from build123d import *

# Parameters (mm, degrees)
F1_DEPTH  = 6.35
F2_R      = 46.355
F2_R_2    = 8.1788
F2_R_3    = 10.16
F2_R_4    = 3.175
F2_R_5    = 3.556
F2_R_6    = 2.38125
F3_DEPTH  = 6.351
F4_R      = 48.895
F5_DEPTH  = 2.413
F6_SIZE   = 0.79375
F7_R      = 6.731
F7_R_2    = 7.1501
F8_DEPTH  = 3.96875
F9_R      = 3.571875
F10_DEPTH = 6.351
F11_R     = 6.746875
F12_DEPTH = 3.96875


with BuildPart() as f1:
    # F0 (on Top) → F1 (new body)
    with BuildSketch(Plane.XY):
        with BuildLine():
            ThreePointArc((152.4, 107.95), (150.540128, 112.440128), (146.05, 114.3))
            Line((146.05, 114.3), (-146.05, 114.3))
            ThreePointArc((-146.05, 114.3), (-150.540128, 112.440128), (-152.4, 107.95))
            Line((-152.4, 107.95), (-152.4, -107.95))
            ThreePointArc((-152.4, -107.95), (-150.540128, -112.440128), (-146.05, -114.3))
            Line((-146.05, -114.3), (146.05, -114.3))
            ThreePointArc((146.05, -114.3), (150.540128, -112.440128), (152.4, -107.95))
            Line((152.4, -107.95), (152.4, 107.95))
        make_face()
    extrude(amount=F1_DEPTH)

    # F2 (on face) → F3 (cut, through all)
    with BuildSketch(Plane(origin=(0, 0, 0), x_dir=(1, 0, 0), z_dir=(0, 0, -1))):
        Circle(F2_R)
        with Locations((60.325, 0)):
            Circle(F2_R_2)
        with Locations((53.975, 38.1)):
            Circle(F2_R_3)
        with Locations((54.305205, -31.353125)):
            Circle(F2_R_4)
        with Locations((-54.305205, 31.353125)):
            Circle(F2_R_4)
        with Locations((25.4, 54.900886)):
            Circle(F2_R_5)
        with Locations((-60.245562, -5.453398)):
            Circle(F2_R_5)
        with Locations((39.444204, -55.973177)):
            Circle(F2_R_5)
        with Locations((108.331, 106.68)):
            Circle(F2_R_6)
        with Locations((-108.331, 106.68)):
            Circle(F2_R_6)
        with Locations((-108.331, -106.68)):
            Circle(F2_R_6)
        with Locations((108.331, -106.68)):
            Circle(F2_R_6)
    extrude(amount=-F3_DEPTH, mode=Mode.SUBTRACT)

    # F4 (on face) → F5 (cut)
    with BuildSketch(Plane(origin=(0, 0, 0), x_dir=(1, 0, 0), z_dir=(0, 0, -1))):
        Circle(F4_R)
    extrude(amount=-F5_DEPTH, mode=Mode.SUBTRACT)

    # F6
    f6_edges = [f1.edges().sort_by_distance(p)[0] for p in [
        (-46.355, 0, 2.413),
    ]]
    chamfer(f6_edges, length=F6_SIZE)

    # F7 (on face) → F8 (cut)
    with BuildSketch(Plane(origin=(0, 0, 0), x_dir=(1, 0, 0), z_dir=(0, 0, -1))):
        with Locations((39.444204, -55.973177)):
            Circle(F7_R)
        with Locations((-60.245562, -5.453398)):
            Circle(F7_R_2)
        with Locations((25.4, 54.900886)):
            Circle(F7_R)
    extrude(amount=-F8_DEPTH, mode=Mode.SUBTRACT)

    # F9 (on face) → F10 (cut, through all)
    with BuildSketch(Plane(origin=(0, 0, 0), x_dir=(1, 0, 0), z_dir=(0, 0, -1))):
        with Locations((56.136862, 18.239972)):
            Circle(F9_R)
        with Locations((-12.272152, -57.735935)):
            Circle(F9_R)
        with Locations((-43.86471, 39.495963)):
            Circle(F9_R)
    extrude(amount=-F10_DEPTH, mode=Mode.SUBTRACT)

    # F11 (on face) → F12 (cut)
    with BuildSketch(Plane(origin=(0, 0, 0), x_dir=(1, 0, 0), z_dir=(0, 0, -1))):
        with Locations((-12.272152, -57.735935)):
            Circle(F11_R)
        with Locations((56.136862, 18.239972)):
            Circle(F11_R)
        with Locations((-43.86471, 39.495963)):
            Circle(F11_R)
    extrude(amount=-F12_DEPTH, mode=Mode.SUBTRACT)


solid = f1.part
Geometry check sheet. Reference: the model listing, model coordinates, mm. A direction names the side the tool comes from. Coordinates: 2 decimals unless noted, no trailing zeros. Order: outer loops, then holes, each group sorted by start corner. A loop starts at its lowest first (then second) coordinate and runs counter-clockwise, first axis right, second up. Notation, with made-up numbers: (59, -25) -> (78, -25) arc R10 cw to (78, -20) -> close; hole circle Ø3 at (60, 19). An arc over 180 degrees is marked (long way). Use a Markdown table: item, result. Add a question column.
1. Material ranges on L1, parallel to X at y = 106.68, z = 3.75; L2, parallel to X at y = -18, z = 4.25; L3, parallel to Y at x = 0, z = 1.8 (3 decimals), recorded low to high.
2. Go/stop test with a flat-tipped pin: pin 1 Ø10 at (x, y) = (60.325, 0) entering from +Z. Record where the tip stops, or that it passes through.
3. Cross-section at A-A (x = 0). Enter the section's corners in (y, z) (3 decimals), and give its area (3 significant figures).
4. Mould release check, pull along Y, two halves, no side actions. Record for faces 3 (the face through (2, 114.3, 3)), 4 (the face through (-13.15, 51.046, 1.957)), 5 (the face through (-152.4, 2, 3)): pulls with the +Y half, pulls with the -Y half, needs draft (parallel to the pull), parting line crosses it, or undercut.
5. Set-up check for faces 1 (the face through (42, 59, 3.969)), 2 (the face through (42.8, 17.8, 4.8)): record each of +Z, -Z, +X, -X, +Y, -Y from which the full face is reachable in a straight line by a thin tool's end or side.
6. Cross-section at B-B (z = 5). Give the number of separate pieces and of enclosed holes in the cut face, and give its area (3 significant figures).
Filled sheet:
| question | item | result |
|---|---|---|
| 1 | L1 | -152.4 to -110.71, -105.95 to 105.95, 110.71 to 152.4 |
| 1 | L2 | -152.4 to -42.72, 42.72 to 52.57, 59.7 to 152.4 |
| 1 | L3 | -114.3 to -48.895, 48.895 to 114.3 |
| 2 | pin 1 | through |
| 3 | outline | (-114.3, 0) -> (-48.895, 0) -> (-48.895, 2.413) -> (-47.149, 2.413) -> (-46.355, 3.207) -> (-46.355, 6.35) -> (-114.3, 6.35) -> close; (46.355, 3.207) -> (47.149, 2.413) -> (48.895, 2.413) -> (48.895, 0) -> (114.3, 0) -> (114.3, 6.35) -> (46.355, 6.35) -> close |
| 3 | area | 850 mm2 |
| 4 | face 3 | pulls with the +Y half |
| 4 | face 4 | undercut |
| 4 | face 5 | needs draft |
| 5 | face 1 | -Z |
| 5 | face 2 | +Z, -Z |
| 6 | separate pieces | 1 |
| 6 | enclosed holes | 15 |
| 6 | area | 62,000 mm2 |
